Part model, mm, in its own coordinate system. A direction names the side the tool comes from. Coordinates: 2 decimals unless noted, no trailing zeros. Order: outer loops, then holes, each group sorted by start corner. A loop starts at its lowest first (then second) coordinate and runs counter-clockwise, first axis right, second up. Notation, with made-up numbers: (37, 50) - (55, 50) arc R15 cw to (55, 75) - close; hole circle Ø1 at (-12, 41). An arc over 180 degrees is marked (long way). Use a Markdown table: item, result. Add a question column.
1) Two-plate mould, pull along Y, no slides. Class faces 1 (the face through (8160, 1350, 246)), 2 (the face through (7450, 1177, 1896)), 3 (the face through (8677, 450, 796)), 4 (the face through (7830, 1000, 1095)): +Y half, -Y half, draft (parallel to the pull), parting line (faces both ways), or undercut.
2) Tool access for faces 5 (the face through (8850, 906, 1346)), 6 (the face through (8677, 450, 1896)), 7 (the face through (7450, 1177, 1346)): list every direction of +Z, -Z, +X, -X, +Y, -Y with a clear straight run to the whole face (end or side of a thin tool).
3) Drop flat-ended pins along their axis: P1, Ø3, axis at x = 8192.5, y = 1209, coming from the -Z side; P2, Ø4, axis at y = 737.5, z = 1810, coming from the -X side; P3, Ø6, axis at x = 7696, z = 1052, coming from the -Y side. Give the stop position or say it passes through.
4) Saw through at A-A on x = 8597.5. List the corners of the cut face in (y, z).
5) Wall check: L1, parallel to Z at x = 8767, y = 979; L2, parallel to X at y = 1024, z = 1781.5; L3, parallel to Y at x = 8811, z = 181.5. Give the ranges that are in metal, low to high. Write a range as [from, to].
6) Saw through at C-C on z = 891.5. List the corners of the cut face in (x, y), then the cut area to 4 significant figures.
7) Saw through at D-D on y = 637.5. List the corners of the cut face in (x, z).
8) Saw through at B-B on y = 1102.5. List the corners of the cut face in (x, z), then the cut area to 3 significant figures.
```python
from build123d import *

# Parameters (mm, degrees)
BOX3529_W        = 1400
BOX3529_H        = 900
BOX3529_DEPTH    = 500
ARRAY281_Z_COUNT = 4
ARRAY281_Z_PITCH = 550
BOX3527_W        = 400
BOX3527_H        = 600
BOX3527_DEPTH    = 2200
BOX3528_W        = 1500
BOX3528_H        = 400
BOX3528_DEPTH    = 2200


with BuildPart() as array281:
    # Box3529 → Box3529 (new body)
    with BuildSketch(Plane(origin=(8850, 1350, 0), x_dir=(-1, 0, 0), z_dir=(0, 0, 1))):
        with Locations((700, 450)):
            Rectangle(BOX3529_W, BOX3529_H)
    extrude(amount=BOX3529_DEPTH)

    # Array281 Z: Array281 ×4


with BuildPart() as array281_1:
    add(array281.part)
    with Locations(*[(0, 0, i * ARRAY281_Z_PITCH) for i in range(1, ARRAY281_Z_COUNT)]):
        add(array281.part)


with BuildPart() as box3527:
    # Box3527 → Box3527 (new body)
    with BuildSketch(Plane(origin=(8900, 1000, 0), x_dir=(-1, 0, 0), z_dir=(0, 0, 1))):
        with Locations((200, 300)):
            Rectangle(BOX3527_W, BOX3527_H)
    extrude(amount=BOX3527_DEPTH)


with BuildPart() as cut003:
    # Box3528 → Box3528 (new body)
    with BuildSketch(Plane(origin=(8900, 1400, 0), x_dir=(-1, 0, 0), z_dir=(0, 0, 1))):
        with Locations((750, 200)):
            Rectangle(BOX3528_W, BOX3528_H)
    extrude(amount=BOX3528_DEPTH)

    # Fusion015: union Box3527
    add(box3527.part)

    # Cut003: cut Array281
    add(array281_1.part, mode=Mode.SUBTRACT)


solid = cut003.part
```
Results are:
| question | item | result |
|---|---|---|
| 1 | face 1 | undercut |
| 1 | face 2 | draft |
| 1 | face 3 | undercut |
| 1 | face 4 | -Y half |
| 2 | face 5 | none |
| 2 | face 6 | -X |
| 2 | face 7 | -Y |
| 3 | P1 | z = 500 |
| 3 | P2 | x = 8850 |
| 3 | P3 | y = 1000 |
| 4 | outline | (400, 0) - (450, 0) - (450, 500) - (1350, 500) - (1350, 0) - (1400, 0) - (1400, 2200) - (400, 2200) - close; hole (450, 550) - (1350, 550) - (1350, 1050) - (450, 1050) - close; hole (450, 1100) - (1350, 1100) - (1350, 1600) - (450, 1600) - close; hole (450, 1650) - (1350, 1650) - (1350, 2150) - (450, 2150) - close |
| 5 | L1 | [500, 550], [1050, 1100], [1600, 1650], [2150, 2200] |
| 5 | L2 | [7400, 7450], [8850, 8900] |
| 5 | L3 | [400, 450], [1350, 1400] |
| 6 | outline | (7400, 1000) - (7450, 1000) - (7450, 1350) - (8850, 1350) - (8850, 450) - (8500, 450) - (8500, 400) - (8900, 400) - (8900, 1400) - (7400, 1400) - close |
| 6 | area | 157,500 mm2 |
| 7 | outline | (8500, 500) - (8850, 500) - (8850, 0) - (8900, 0) - (8900, 2200) - (8500, 2200) - (8500, 2150) - (8850, 2150) - (8850, 1650) - (8500, 1650) - (8500, 1600) - (8850, 1600) - (8850, 1100) - (8500, 1100) - (8500, 1050) - (8850, 1050) - (8850, 550) - (8500, 550) - close |
| 8 | outline | (7400, 0) - (7450, 0) - (7450, 500) - (8850, 500) - (8850, 0) - (8900, 0) - (8900, 2200) - (7400, 2200) - close; hole (7450, 550) - (8850, 550) - (8850, 1050) - (7450, 1050) - close; hole (7450, 1100) - (8850, 1100) - (8850, 1600) - (7450, 1600) - close; hole (7450, 1650) - (8850, 1650) - (8850, 2150) - (7450, 2150) - close |
| 8 | area | 500,000 mm2 |
